Input: part model. Units: mm. Frame: model coordinates. A direction names the side the tool comes from. Give positions to 0.01 mm unless a question says otherwise; leave off trailing zeros. Loops run counter-clockwise (first coordinate to the right, second up) from the corner with the lowest first, then second, coordinate; pieces in that order, holes last. Notation, with made-up numbers: M 65,-19.5 L 104,-19.5 A13 ccw 104,-6.5 Z; hole C 54,33.5 d1. An arc over 180 degrees is marked long. Answer as a JSON object with one key per item and string values. Group by question number.
```python
from build123d import *

# Parameters (mm, degrees)
PLATE_SKETCH_W            = 200
PLATE_SKETCH_H            = 70
PLATE_EXTRUDE_DEPTH       = 15
HINGE_PLATE_EXTRUDE_DEPTH = 10
PIN_SKETCH_R              = 5.5
UPPER_PIN_EXTRUDE_DEPTH   = 25
LOWER_START               = -45
PIN_SKETCH_2_R            = 5.5
LOWER_PIN_EXTRUDE_DEPTH   = 25


with BuildPart() as part:
    # Plate Sketch → Plate Extrude (new body)
    with BuildSketch(Plane.XY):
        Rectangle(PLATE_SKETCH_W, PLATE_SKETCH_H)
    extrude(amount=-PLATE_EXTRUDE_DEPTH)

    # Hinge Plate Sketch → Hinge Plate Extrude (add, symmetric)
    with BuildSketch(Plane(origin=(0, 0, 0), x_dir=(1, 0, 0), z_dir=(0, 1, 0))):
        with BuildLine():
            Line((100, 15), (107.5, 15))
            ThreePointArc((107.5, 15), (115, 7.5), (107.5, 0))
            Line((107.5, 0), (100, 0))
            Line((100, 0), (100, 15))
        make_face()
    hinge_plate_extrude = extrude(amount=HINGE_PLATE_EXTRUDE_DEPTH, both=True)

    # Pin Sketch → Upper Pin Extrude (add)
    with BuildSketch(Plane(origin=(0, 10, 0), x_dir=(1, 0, 0), z_dir=(0, 1, 0))):
        with Locations(Location((107.5, 7.5, 0), (0, 0, 270))):
            Circle(PIN_SKETCH_R)
    upper_pin_extrude = extrude(amount=UPPER_PIN_EXTRUDE_DEPTH)

    # Pin Sketch<2> → Lower Pin Extrude (add)
    with BuildSketch(Plane(origin=(0, 10, 0), x_dir=(1, 0, 0), z_dir=(0, 1, 0)).offset(LOWER_START)):
        with Locations(Location((107.5, 7.5, 0), (0, 0, 270))):
            Circle(PIN_SKETCH_2_R)
    lower_pin_extrude = extrude(amount=LOWER_PIN_EXTRUDE_DEPTH)

    # Hinge Mirror: Hinge Plate Extrude, Upper Pin Extrude, Lower Pin Extrude across plane
    add(hinge_plate_extrude.mirror(Plane(origin=(0, 0, 0), x_dir=(0, 0, 1), z_dir=(1, 0, 0))))
    add(upper_pin_extrude.mirror(Plane(origin=(0, 0, 0), x_dir=(0, 0, 1), z_dir=(1, 0, 0))))
    add(lower_pin_extrude.mirror(Plane(origin=(0, 0, 0), x_dir=(0, 0, 1), z_dir=(1, 0, 0))))


solid = part.part
```
1. Mould query, pull axis X, two halves, no side actions, for faces 1 (the cylindrical face through (-115, 0.14, -7.66)), 2 (the flat face through (-100, 22, -7)), 3 (the flat face through (-1, -35, -7)). Classes: pulls with the +X half, pulls with the -X half, needs draft (parallel to the pull), parting line crosses it, or undercut.
2. First-contact query: P1, Ø6, axis at y = 26.5, z = -9.5, coming from the +X side; P2, Ø12, axis at x = 21.5, y = -14.5, coming from the +Z side; P3, Ø1.5, axis at y = -13, z = -4.5, coming from the +X side; P4, Ø4.5, axis at y = 22, z = -10, coming from the -X side. Flat tips, straight axial feed; report the tip coordinate or a pass-through.
3. Section B-B (z = -7.5). Output: boundary loops of the cut face in (x, y), then the cut area to 3 significant figures.
4. Section A-A (y = 28.5). Output: boundary loops of the cut face in (x, z), then the cut area to 3 significant figures.
5. Material intervals for L1, parallel to X at y = 27.5, z = -7.5; L2, parallel to X at y = -17.5, z = -9.75; L3, parallel to X at y = 12, z = -14.5, sorted ascending.
6. Reachability of faces 4 (the cylindrical face through (112.953, 22.325, -8.216)), 5 (the cylindrical face through (-112.953, -22.675, -8.216)), 6 (the flat face through (100, 22, -7)) from +Z, -Z, +X, -X, +Y, -Y: full face, straight path, thin tool, end or side. Return the list, or none.
Geometry results:
{
 "1": {"face 1": "pulls with the -X half", "face 2": "undercut", "face 3": "needs draft"},
 "2": {"P1": "x = 113", "P2": "z = 0", "P3": "x = 112.52", "P4": "x = -112.99"},
 "3": {"outline": "M -115,-10 L -113,-10 L -113,-35 L -102,-35 L -102,-10 L -100,-10 L -100,-35 L 100,-35 L 100,-10 L 102,-10 L 102,-35 L 113,-35 L 113,-10 L 115,-10 L 115,10 L 113,10 L 113,35 L 102,35 L 102,10 L 100,10 L 100,35 L -100,35 L -100,10 L -102,10 L -102,35 L -113,35 L -113,10 L -115,10 Z", "area": "15,700 mm2"},
 "4": {"outline": "C -107.5,-7.5 d11; M -100,-15 L 100,-15 L 100,0 L -100,0 Z; C 107.5,-7.5 d11", "area": "3,190 mm2"},
 "5": {"L1": "-113 to -102, -100 to 100, 102 to 113", "L2": "-112.52 to -102.48, -100 to 100, 102.48 to 112.52", "L3": "-100 to 100"},
 "6": {"face 4": "+Y", "face 5": "-Y", "face 6": "+Z, -Z, +Y"}
}
